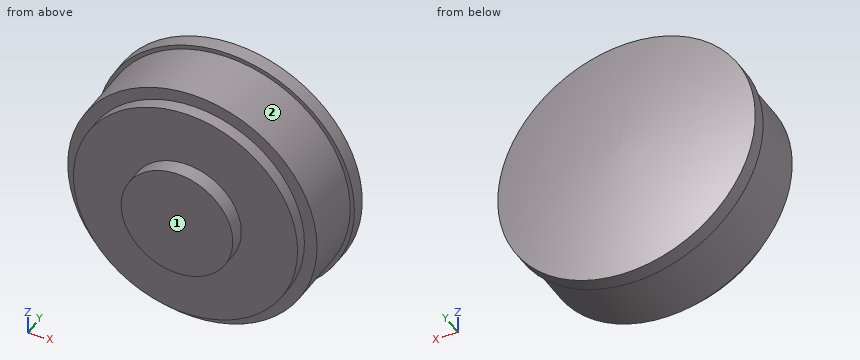
Autodesk Inventor part; units mm, degrees
ref_plane "YZ Plane" through (0, 0, 0) normal (1, 0, 0) x (0, 1, 0)
ref_plane "XZ Plane" through (0, 0, 0) normal (0, 1, 0) x (-1, 0, 0)
ref_plane "XY Plane" through (0, 0, 0) normal (0, 0, 1) x (1, 0, 0)
sketch "Sketch1" plane through (0, 0, 0) normal (0, 1, 0) x (-1, 0, 0)
  circle A0 centre (0, 0) radius 19
  dimension "d0" = 38
extrude "Extrusion1" add sketch "Sketch1" along normal blind 5.4
sketch "Sketch2" plane through (0, 5.4, 0) normal (0, 1, 0) x (1, 0, 0)
  circle A0 centre (0, 0) radius 38.125
  dimension "d3" = 76.25
extrude "Extrusion2" add sketch "Sketch2" along normal blind 4.35
sketch "Sketch3" plane through (0, 9.75, 0) normal (0, 1, 0) x (1, 0, 0)
  circle A0 centre (0, 0) radius 42.4
  dimension "d6" = 84.8
extrude "Extrusion3" add sketch "Sketch3" along normal blind 21
sketch "Sketch4" plane through (0, 30.75, 0) normal (0, 1, 0) x (1, 0, 0)
  circle A0 centre (0, 0) radius 43.8
  dimension "d9" = 87.6
extrude "Extrusion4" add sketch "Sketch4" along normal blind 5
sketch "Sketch5" plane through (0, 0, 0) normal (1, 0, 0) x (0, 1, 0)
  line L0 (35.75, -43.8) -> (35.75, 43.8)
  line L1 (35.75, -43.8) -> (35.75, 43.8)
  line L2 (30.75, -43.8) -> (30.75, 43.8)
  line L3 (35.75, -43.8) -> (35.75, 43.8)
  line L4 (30.75, -43.8) -> (30.75, 43.8)
  line L5 (35.75, 0) -> (40.75, 0)
  arc A0 (40.75, 0) -> (35.75, 43.8) centre (-179.7193, -2.9823) ccw
  line L6 (35.75, 0) -> (35.75, 43.8)
  point P0 (0, 0)
  dimension "d12" = 5
revolve "Revolution1" add sketch "Sketch5" angle 360 about axis through (0, 35.75, 0) along (0, 1, 0)
properties part number "N95 Filter"
Here's how the part is built. I have some questions about the finished solid (model axes, mm). Face numbers are marked on the shaded views. A direction names the side the tool comes from. Round coordinates to 2 decimals unless told otherwise and drop trailing zeros. Write each question's results on one line, items separated by ' | '. Start each with the question number.
(1) On a 3-axis mill with a long thin cutter (end or side, diameter ignored), from which of +Z, -Z, +X, -X, +Y, -Y can I reach the whole of each face in a straight line? I mean the marked faces 1 and 2. Say none if no direction works.
(2) If I drill on probe 1 along Y at (x, z) = (1, 0.5); probe 2 along Z at (x, y) = (33, 16); probe 3 along Y at (x, z) = (8.5, -39.5), over which ranges is the centre line in solid material (lowest first)? Write a range as from..to.
(3) Will these pins go through, and if not, where does the flat tip stop? P1, Ø10, axis at x = -23, y = 34, coming from the +Z side; P2, Ø10, axis at x = 9, y = 22, coming from the -Z side; P3, Ø8, axis at x = -9.5, y = 4.5, coming from the +Z side.
Solved:
1) face 1: +Z, -Z, +X, -X, -Y | face 2: -Y
2) probe 1: y = 0..40.73 | probe 2: z = -26.62..26.62 | probe 3: y = 9.75..36.46
3) P1: stops at z = 39.93 | P2: stops at z = -42.21 | P3: stops at z = 37.71
